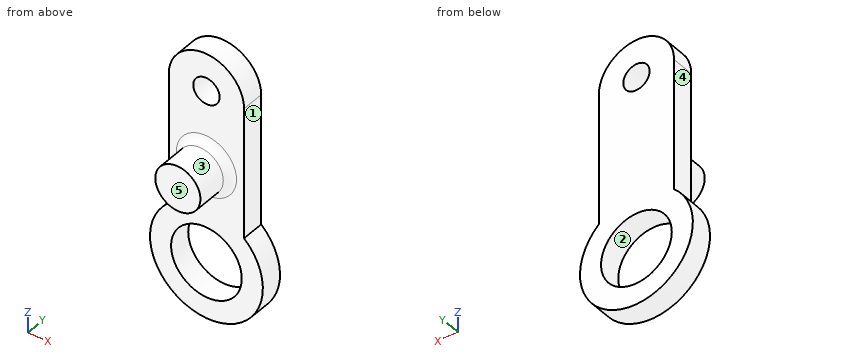
Autodesk Inventor part; units mm, degrees
ref_plane "工作平面2" through (0, 2.2, 0) normal (0, 1, 0) x (-1, 0, 0)
ref_plane "YZ Plane" through (0, 0, 0) normal (1, 0, 0) x (0, 1, 0)
ref_plane "XY Plane" through (0, 0, 0) normal (0, 0, 1) x (1, 0, 0)
sketch "草圖1" plane through (0, 0, 0) normal (0, 1, 0) x (-1, 0, 0)
  circle A0 centre (0, 0) radius 1.75
  arc A1 (5, 0) -> (-5, 0) centre (0, 0) ccw
  circle A2 centre (0, -23) radius 4.7
  arc A3 (-5, -17.4098) -> (5, -17.4098) centre (0, -23) ccw
  line L0 (-5, 0) -> (-5, -17.4098)
  line L1 (5, 0) -> (5, -17.4098)
  line L2 (0, 0) -> (0, -1.75) construction
  line L3 (0, -15.5) -> (0, -23) construction
  dimension "d0" = 3.5
  dimension "d1" = 10
  dimension "d2" = 23
  dimension "d3" = 9.4
  dimension "d4" = 15
extrude "擠出1" add sketch "草圖1" along normal blind 3
ref_plane "工作平面2" through (0, 2.2, 0) normal (0, 1, 0) x (-1, 0, 0)
sketch "草圖3" plane through (0, 2.2, 0) normal (0, 1, 0) x (-1, 0, 0)
  circle A0 centre (0, -23) radius 4.7
  circle A1 centre (0, 0) radius 1.75
  line L0 (-5, 0) -> (-5, -17.4098)
  arc A2 (-5, -17.4098) -> (5, -17.4098) centre (0, -23) ccw
  line L1 (5, -17.4098) -> (5, 0)
  arc A3 (5, 0) -> (-5, 0) centre (0, 0) ccw
sketch "草圖4" plane through (0, 0, 0) normal (0, -1, 0) x (1, 0, 0)
  line L0 (0, 0) -> (0, -10) construction
  circle A0 centre (0, -10) radius 3
  dimension "d13" = 10
  dimension "d14" = 6
extrude "擠出3" add sketch "草圖4" along normal blind 5
fillet "圓角1" radius 1 1 edges at (-3, 0, -10)
properties part number "轉軸" material "ABS Plastic"
Part model, mm, in its own coordinate system. Face numbers are marked on the shaded views. A direction names the side the tool comes from. Give positions to 0.01 mm unless a question says otherwise; leave off trailing zeros. Loops run counter-clockwise (first coordinate to the right, second up) from the corner with the lowest first, then second, coordinate; pieces in that order, holes last. Notation, with made-up numbers: M 20,88 L 37,88 A13 cw 37,98 Z; hole C 19,-33.75 d2. An arc over 180 degrees is marked long. Put each result on its own line as item: value. Start each with the question number.
1) Saw through at A-A (x = 0). List the corners of the cut face in (y, z).
2) Flat gauge pins, fed straight in: pin 1 (5.5 mm diameter, centred on x = 0, z = 0, fed in from +Y); pin 2 (2.5 mm diameter, centred on y = 2, z = -11.5, fed in from -X); pin 3 (0.9 mm diameter, centred on y = 1, z = -11, fed in from +X); pin 4 (2 mm diameter, centred on x = -5.5, z = -9.5, fed in from -Y). Where does each tip first touch, or does it go through?
3) Probe probe 1 along Z at (x, y) = (0, 2.35); probe 2 along Y at (x, z) = (1.75, -29); probe 3 along Z at (x, y) = (0.75, 2.75). List the from-to ranges inside material, lowest first.
4) Pull direction X, two halves, no side cores. Call the marked faces 1, 2 and 3: +X half, -X half, draft (parallel to the pull), parting line (faces both ways), or undercut.
5) Saw through at C-C (z = -23.5). List the corners of the cut face in (x, y), then the cut area to 3 significant figures.
6) Saw through at B-B (y = 1). List the corners of the cut face in (x, z), then the cut area to 3 significant figures.
7) Saw through at D-D (z = -10). List the corners of the cut face in (x, y).
8) 3-axis set-ups, long thin cutter, end or side, ignore diameter. For the marked faces 4 and 5: which of +Z, -Z, +X, -X, +Y, -Y reach the whole face in a straight line?
Numbers:
1. outline: M -5,-13 L -1,-13 A1 cw 0,-14 L 0,-18.3 L 3,-18.3 L 3,-1.75 L 0,-1.75 L 0,-6 A1 cw -1,-7 L -5,-7 Z; M 0,-30.5 L 3,-30.5 L 3,-27.7 L 0,-27.7 Z; M 0,1.75 L 3,1.75 L 3,5 L 0,5 Z
2. pin 1: y = 3
2. pin 2: x = -5
2. pin 3: x = 5
2. pin 4: y = 0
3. probe 1: -30.5 to -27.7, -18.3 to -1.75, 1.75 to 5
3. probe 2: 0 to 3
3. probe 3: -30.46 to -27.64, -18.36 to -1.58, 1.58 to 4.94
4. face 1: +X half
4. face 2: undercut
4. face 3: parting line
5. outline: M -7.48,0 L -4.67,0 L -4.67,3 L -7.48,3 Z; M 4.67,0 L 7.48,0 L 7.48,3 L 4.67,3 Z
5. area: 16.9 mm^2
6. outline: M -5,-17.41 A7.5 ccw long 5,-17.41 L 5,0 A5 ccw -5,0 Z; hole C 0,-23 d9.4; hole C 0,0 d3.5
6. area: 298 mm^2
7. outline: M -5,0 L -4,0 A1 cw -3,-1 L -3,-5 L 3,-5 L 3,-1 A1 cw 4,0 L 5,0 L 5,3 L -5,3 Z
8. face 4: +Z, -X, +Y, -Y
8. face 5: +Z, -Z, +X, -X, -Y
